Part model, mm, in its own coordinate system. Give positions to 0.01 mm unless a question says otherwise; leave off trailing zeros. Order: outer loops, then holes, each group sorted by start corner. A loop starts at its lowest first (then second) coordinate and runs counter-clockwise, first axis right, second up. Notation, with made-up numbers: (-39.5, 35.25) - (-31.5, 35.25) arc R10 ccw to (-31.5, 46.25) - close; hole circle Ø1 at (-2, 20.25). An arc over 180 degrees is marked (long way). Use a Markdown table: item, result. Add a question column.
from build123d import *

# Parameters (mm, degrees)
SKETCH1_W              = 900
SKETCH1_H              = 200
SKETCH1_R              = 5
BOSS_EXTRUDE1_DEPTH    = 15
SKETCH2_W              = 208
SKETCH2_H              = 126
SHREDDER_OPENING_DEPTH = 16
SKETCH3_W              = 170
SKETCH3_H              = 76.5
SKETCH3_R              = 5
LEGS_ADD_ON_DEPTH      = 15


with BuildPart() as part:
    # Sketch1 → Boss-Extrude1 (new body)
    with BuildSketch(Plane(origin=(0, 0, 0), x_dir=(1, 0, 0), z_dir=(0, 1, 0))):
        Rectangle(SKETCH1_W, SKETCH1_H)
        with Locations((425, -75)):
            Circle(SKETCH1_R, mode=Mode.SUBTRACT)
        with Locations((425, 75)):
            Circle(SKETCH1_R, mode=Mode.SUBTRACT)
        with Locations((-425, -75)):
            Circle(SKETCH1_R, mode=Mode.SUBTRACT)
        with Locations((-425, 75)):
            Circle(SKETCH1_R, mode=Mode.SUBTRACT)
    extrude(amount=-BOSS_EXTRUDE1_DEPTH)

    # Sketch2 → Shredder Opening (cut, through all)
    with BuildSketch(Plane.XZ.offset(15)):
        with Locations((-275, 7.5)):
            Rectangle(SKETCH2_W, SKETCH2_H)
    extrude(amount=-SHREDDER_OPENING_DEPTH, mode=Mode.SUBTRACT)

    # Sketch3 → Legs add on (add, through all)
    with BuildSketch(Plane(origin=(0, 0, 0), x_dir=(1, 0, 0), z_dir=(0, 1, 0))):
        with Locations((115, 138.25)):
            Rectangle(SKETCH3_W, SKETCH3_H)
        with Locations((175, 151.5)):
            Circle(SKETCH3_R, mode=Mode.SUBTRACT)
        with Locations((55, 151.5)):
            Circle(SKETCH3_R, mode=Mode.SUBTRACT)
    extrude(amount=-LEGS_ADD_ON_DEPTH)


solid = part.part
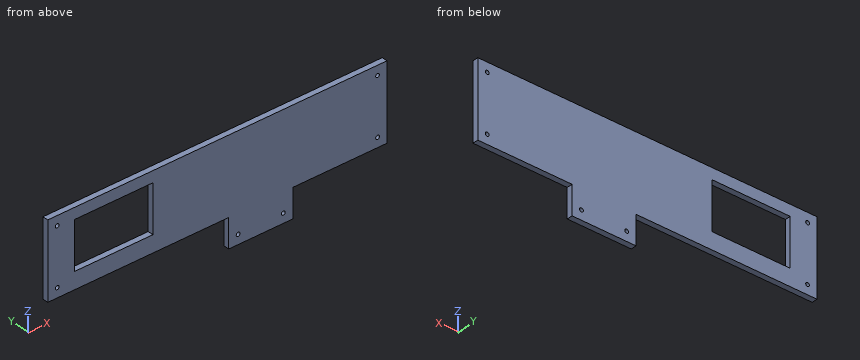
1. Cut at A-A (x = -354). Write the cut outline in (y, z).
2. Cut at C-C (z = -108). Write the cut outline in (x, y), plus the area to 3 significant figures.
3. Pin check, flat tips, straight feed: P1, Ø13, axis at x = -425, z = 75, coming from the +Y side; P2, Ø4, axis at y = -13.5, z = -114.5, coming from the -X side; P3, Ø7.5, axis at x = -284, y = -11, coming from the -Z side; P4, Ø8, axis at y = -6.5, z = -135.5, coming from the +X side. Stop position of each tip, or through.
4. Drill centre lines: probe 1 along X at (y, z) = (-11.5, -151.5); probe 2 along Z at (x, y) = (425, -10.75); probe 3 along Z at (x, y) = (175, -8). Where is each one in solid material? Low to high. Write a range as [from, to].
5. Cut at D-D (x = 228). Write the cut outline in (y, z).
6. Cut at B-B (y = -8.25). Write the cut outline in (x, z), plus the area to 3 significant figures.
Responses:
| question | item | result |
|---|---|---|
| 1 | outline | (-15, -100) - (0, -100) - (0, -55.5) - (-15, -55.5) - close; (-15, 70.5) - (0, 70.5) - (0, 100) - (-15, 100) - close |
| 2 | outline | (30, -15) - (200, -15) - (200, 0) - (30, 0) - close |
| 2 | area | 2,550 mm² |
| 3 | P1 | stops at y = 0 |
| 3 | P2 | stops at x = 30 |
| 3 | P3 | stops at z = -100 |
| 3 | P4 | stops at x = 200 |
| 4 | probe 1 | x = [30, 50], [60, 170], [180, 200] |
| 4 | probe 2 | z = [-100, -80], [-70, 70], [80, 100] |
| 4 | probe 3 | z = [-176.5, -156.5], [-146.5, 100] |
| 5 | outline | (-15, -100) - (0, -100) - (0, 100) - (-15, 100) - close |
| 6 | outline | (-450, -100) - (30, -100) - (30, -176.5) - (200, -176.5) - (200, -100) - (450, -100) - (450, 100) - (-450, 100) - close; hole circle Ø10 at (-425, -75); hole circle Ø10 at (-425, 75); hole (-379, -55.5) - (-171, -55.5) - (-171, 70.5) - (-379, 70.5) - close; hole circle Ø10 at (55, -151.5); hole circle Ø10 at (175, -151.5); hole circle Ø10 at (425, -75); hole circle Ø10 at (425, 75) |
| 6 | area | 166,000 mm² |
